Check sheet for the drawn part. Datum: minimum x, y, z corner. Units: mm. A direction names the side the tool comes from. Round coordinates to 2 decimals unless told otherwise and drop trailing zeros. Order: outer loops, then holes, each group sorted by start corner. A loop starts at its lowest first (then second) coordinate and runs counter-clockwise, first axis right, second up. Notation, with made-up numbers: (71, 27) -> (117, 27) arc R8 cw to (117, 34) -> close; hole circle Ø7 at (65, 17). An arc over 180 degrees is marked (long way). Answer in a Markdown table with one row per item.
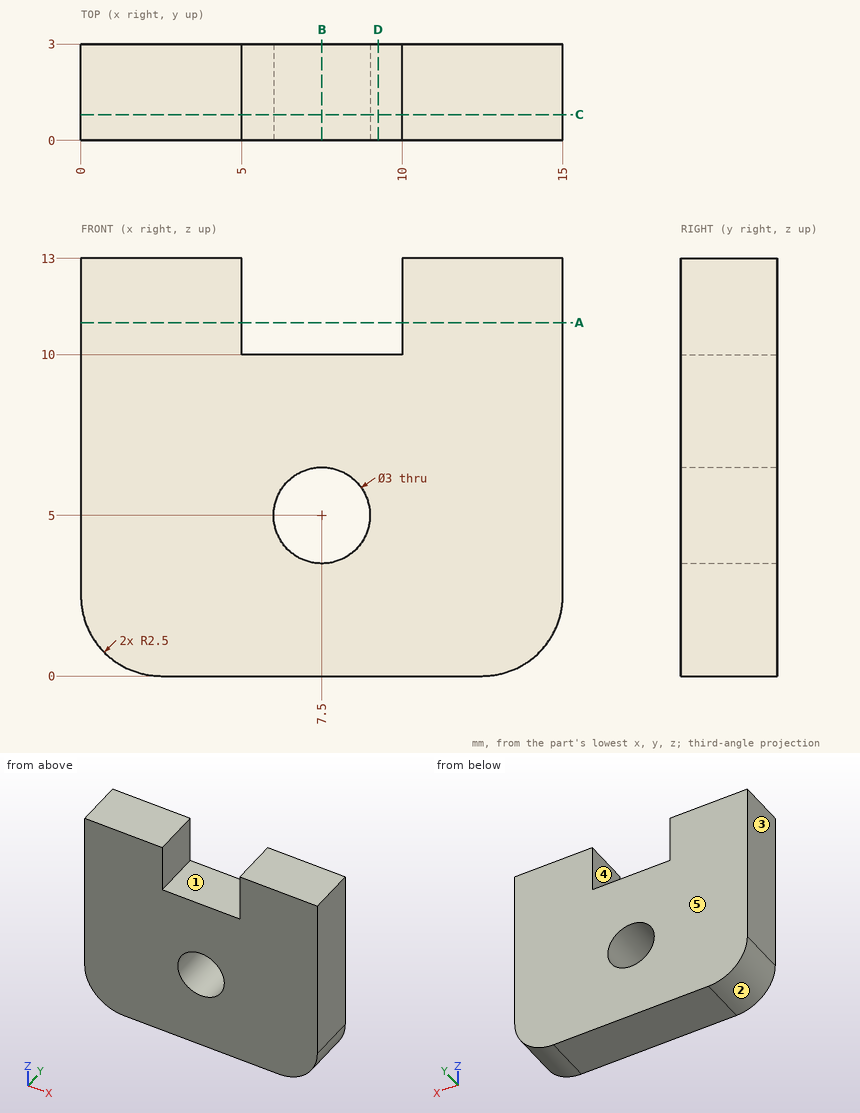
(1) Section check B-B on x = 7.5. Record the boundary of the cut face in (y, z), plus the area to 3 significant figures.
Solutions:
| item | result |
|---|---|
| outline | (0, 0) -> (3, 0) -> (3, 3.5) -> (0, 3.5) -> close; (0, 6.5) -> (3, 6.5) -> (3, 10) -> (0, 10) -> close |
| area | 21.0 mm^2 |
(2) Section check C-C on y = 0.8. Record the boundary of the cut face in (x, z).
Solutions:
| item | result |
|---|---|
| outline | (0, 2.5) arc R2.5 ccw to (2.5, 0) -> (12.5, 0) arc R2.5 ccw to (15, 2.5) -> (15, 13) -> (10, 13) -> (10, 10) -> (5, 10) -> (5, 13) -> (0, 13) -> close; hole circle Ø3 at (7.5, 5) |
(3) Section check D-D on x = 9.25. Record the boundary of the cut face in (y, z), plus the area to 3 significant figures.
Solutions:
| item | result |
|---|---|
| outline | (0, 0) -> (3, 0) -> (3, 10) -> (0, 10) -> close |
| area | 30.0 mm^2 |
(4) Depth check by flat-ended pin: pin 1 Ø0.9 at (x, y) = (8, 1) entering from +Z. Enter the tip coordinate at first touch or a pass-through.
Solutions:
| item | result |
|---|---|
| pin 1 | z = 10 |
(5) Scan lines: probe 1 along X at (y, z) = (0.95, 5); probe 2 along Z at (x, y) = (8, 0.3); probe 3 along Z at (x, y) = (13.25, 2.05). Record each from-to range of solid material in increasing order. Write a range as from..to.
Solutions:
| item | result |
|---|---|
| probe 1 | 0..6, 9..15 |
| probe 2 | 0..3.59, 6.41..10 |
| probe 3 | 0.12..13 |
(6) Tool access check on the marked faces 1 and 2. Record the directions out of +Z, -Z, +X, -X, +Y, -Y that give a thin tool (end or side, any length) a straight path to the whole face; none if there is none.
Solutions:
| item | result |
|---|---|
| face 1 | +Z, +Y, -Y |
| face 2 | -Z, -X, +Y, -Y |
(7) Draft check along X on the marked faces 3, 4 and 5. Enter one of: pulls with the +X half, pulls with the -X half, needs draft (parallel to the pull), parting line crosses it, or undercut.
Solutions:
| item | result |
|---|---|
| face 3 | pulls with the -X half |
| face 4 | undercut |
| face 5 | needs draft |
(8) Section check A-A on z = 11. Record the boundary of the cut face in (x, y), plus the area to 3 significant figures.
Solutions:
| item | result |
|---|---|
| outline | (0, 0) -> (5, 0) -> (5, 3) -> (0, 3) -> close; (10, 0) -> (15, 0) -> (15, 3) -> (10, 3) -> close |
| area | 30.0 mm^2 |
